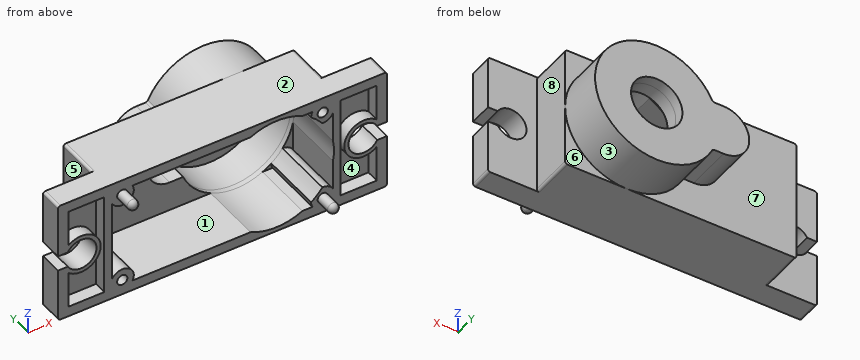
from build123d import *

# Parameters (mm, degrees)
SKETCH1_W            = 22.5
SKETCH1_H            = 12
BOSS_EXTRUDE1_DEPTH  = 6.5
SKETCH2_W            = 22.5
SKETCH2_H            = 12
BOSS_EXTRUDE2_DEPTH  = 0.5
BOSS_EXTRUDE3_DEPTH  = 4.5
SKETCH4_R            = 2.5
BOSS_EXTRUDE4_DEPTH  = 1
CUT_EXTRUDE1_DEPTH   = 7.5
SKETCH6_R            = 3
SKETCH6_R_2          = 2.5
BOSS_EXTRUDE5_DEPTH  = 1.25
BOSS_EXTRUDE7_DEPTH  = 2.25
BOSS_EXTRUDE8_DEPTH  = 1
SKETCH9_R            = 0.625
CUT_EXTRUDE2_DEPTH   = 0.25
SKETCH11_R           = 1.125
SKETCH11_R_2         = 0.5
BOSS_EXTRUDE9_DEPTH  = 6
SKETCH12_R           = 0.5
BOSS_EXTRUDE10_DEPTH = 2
FILLET1_R            = 0.5
FILLET2_R            = 0.25
CUT_EXTRUDE3_DEPTH   = 6


with BuildPart() as part:
    # Sketch1 → Boss-Extrude1 (new body)
    with BuildSketch(Plane(origin=(0, 0, 0), x_dir=(1, 0, 0), z_dir=(0, 1, 0))):
        Rectangle(SKETCH1_W, SKETCH1_H)
        Polygon((10.25, 5), (-10.25, 5), (-10.75, 5), (-10.75, -5), (-10.25, -5), (10.25, -5), (10.75, -5), (10.75, 5), align=None, mode=Mode.SUBTRACT)
    extrude(amount=BOSS_EXTRUDE1_DEPTH)

    # Sketch2 → Boss-Extrude2 (add)
    with BuildSketch(Plane(origin=(0, 6.5, 0), x_dir=(1, 0, 0), z_dir=(0, 1, 0))):
        Rectangle(SKETCH2_W, SKETCH2_H)
    extrude(amount=-BOSS_EXTRUDE2_DEPTH)

    # Sketch3 → Boss-Extrude3 (add)
    with BuildSketch(Plane(origin=(0, 6.5, 0), x_dir=(1, 0, 0), z_dir=(0, 1, 0))):
        with BuildLine():
            Line((-1.25, 2.5), (-0.204356057, 2.5))
            ThreePointArc((-0.204356057, 2.5), (11.25, 0), (-0.204356057, -2.5))
            Line((-0.204356057, -2.5), (-1.25, -2.5))
            ThreePointArc((-1.25, -2.5), (-3.75, 0), (-1.25, 2.5))
        make_face()
        with BuildLine():
            Line((-1.25, 2.1), (0.058661059, 2.1))
            ThreePointArc((0.058661059, 2.1), (10.85, 0), (0.058661059, -2.1))
            Line((0.058661059, -2.1), (-1.25, -2.1))
            ThreePointArc((-1.25, -2.1), (-3.35, 0), (-1.25, 2.1))
        make_face(mode=Mode.SUBTRACT)
    extrude(amount=BOSS_EXTRUDE3_DEPTH)

    # Sketch4 → Boss-Extrude4 (add)
    with BuildSketch(Plane(origin=(0, 11, 0), x_dir=(1, 0, 0), z_dir=(0, 1, 0))):
        with BuildLine():
            ThreePointArc((-1.25, -2.1), (-3.35, 0), (-1.25, 2.1))
            Line((-1.25, 2.1), (0.058661059, 2.1))
            ThreePointArc((0.058661059, 2.1), (10.85, 0), (0.058661059, -2.1))
            Line((0.058661059, -2.1), (-1.25, -2.1))
        make_face()
        with Locations((5.25, 0)):
            Circle(SKETCH4_R, mode=Mode.SUBTRACT)
    extrude(amount=-BOSS_EXTRUDE4_DEPTH)

    # Sketch5 → Cut-Extrude1 (cut, through all)
    with BuildSketch(Plane(origin=(0, 6.5, 0), x_dir=(1, 0, 0), z_dir=(0, 1, 0))):
        with BuildLine():
            Line((-1.25, -2.1), (0.058661059, -2.1))
            ThreePointArc((0.058661059, -2.1), (10.85, 0), (0.058661059, 2.1))
            Line((0.058661059, 2.1), (-1.25, 2.1))
            ThreePointArc((-1.25, 2.1), (-3.35, 0), (-1.25, -2.1))
        make_face()
    extrude(amount=-CUT_EXTRUDE1_DEPTH, mode=Mode.SUBTRACT)

    # Sketch6 → Boss-Extrude5 (add)
    with BuildSketch(Plane.XZ.offset(-10)):
        with Locations((5.25, 0)):
            Circle(SKETCH6_R)
        with Locations((5.25, 0)):
            Circle(SKETCH6_R_2, mode=Mode.SUBTRACT)
    extrude(amount=BOSS_EXTRUDE5_DEPTH)

    # Sketch7 → Boss-Extrude7 (add)
    with BuildSketch(Plane(origin=(0, 0, 0), x_dir=(1, 0, 0), z_dir=(0, 1, 0))):
        with BuildLine():
            Line((-11.25, -6), (-11.25, 6))
            Line((-11.25, 6), (-16, 6))
            Line((-16, 6), (-16, 0.75))
            Line((-16, 0.75), (-15.049038106, 0.75))
            ThreePointArc((-15.049038106, 0.75), (-12.25, 0), (-15.049038106, -0.75))
            Line((-15.049038106, -0.75), (-16, -0.75))
            Line((-16, -0.75), (-16, -6))
            Line((-16, -6), (-11.25, -6))
        make_face()
        with BuildLine():
            Line((-15, 1.430908802), (-15, 5))
            Line((-15, 5), (-11.5, 5))
            Line((-11.5, 5), (-11.5, -5))
            Line((-11.5, -5), (-15, -5))
            Line((-15, -5), (-15, -1.430908802))
            ThreePointArc((-15, -1.430908802), (-11.85, 0), (-15, 1.430908802))
        make_face(mode=Mode.SUBTRACT)
    boss_extrude7 = extrude(amount=BOSS_EXTRUDE7_DEPTH)

    # Sketch8 → Boss-Extrude8 (add)
    with BuildSketch(Plane(origin=(0, 2.25, 0), x_dir=(1, 0, 0), z_dir=(0, 1, 0))):
        with BuildLine():
            Line((-15.049038106, 0.75), (-16, 0.75))
            Line((-16, 0.75), (-16, 6))
            Line((-16, 6), (-11.25, 6))
            Line((-11.25, 6), (-11.25, -6))
            Line((-11.25, -6), (-16, -6))
            Line((-16, -6), (-16, -0.75))
            Line((-16, -0.75), (-15.049038106, -0.75))
            ThreePointArc((-15.049038106, -0.75), (-12.25, 0), (-15.049038106, 0.75))
        make_face()
    boss_extrude8 = extrude(amount=-BOSS_EXTRUDE8_DEPTH)

    # Mirror1: Boss-Extrude7, Boss-Extrude8 across plane
    add(boss_extrude7.mirror(Plane(origin=(0, 0, 0), x_dir=(0, 0, 1), z_dir=(1, 0, 0))))
    add(boss_extrude8.mirror(Plane(origin=(0, 0, 0), x_dir=(0, 0, 1), z_dir=(1, 0, 0))))

    # Sketch9 → Cut-Extrude2 (cut)
    with BuildSketch(Plane.XZ.offset(-10)):
        with Locations((-1.25, 0)):
            Circle(SKETCH9_R)
    extrude(amount=-CUT_EXTRUDE2_DEPTH, mode=Mode.SUBTRACT)

    # Sketch11 → Boss-Extrude9 (add)
    with BuildSketch(Plane.XZ.offset(-6)):
        with Locations((-9.75, 4.5)):
            Circle(SKETCH11_R)
        with Locations((-9.75, -4.5)):
            Circle(SKETCH11_R)
        with Locations((-9.75, -4.5)):
            Circle(SKETCH11_R_2, mode=Mode.SUBTRACT)
        with Locations((9.75, -4.5)):
            Circle(SKETCH11_R)
        with Locations((9.75, 4.5)):
            Circle(SKETCH11_R)
        with Locations((9.75, 4.5)):
            Circle(SKETCH11_R_2, mode=Mode.SUBTRACT)
    extrude(amount=BOSS_EXTRUDE9_DEPTH)

    # Sketch12 → Boss-Extrude10 (add)
    with BuildSketch(Plane.XZ):
        with Locations((-9.75, 4.5)):
            Circle(SKETCH12_R)
        with Locations((9.75, -4.5)):
            Circle(SKETCH12_R)
    extrude(amount=BOSS_EXTRUDE10_DEPTH)

    # Fillet1
    fillet1_edges = [part.edges().sort_by_distance(p)[0] for p in [
        (-10.25, -2, 4.5),
        (9.25, -2, -4.5),
    ]]
    fillet(fillet1_edges, radius=FILLET1_R)

    # Fillet2
    fillet2_edges = [part.edges().sort_by_distance(p)[0] for p in [
        (-16, 1.125, 6),
        (-16, 1.125, -6),
        (16, 1.125, -6),
        (16, 1.125, 6),
        (-0.204356057, 8.75, -2.5),
        (-0.204356057, 8.75, 2.5),
        (-11.25, 4.375, -6),
        (11.25, 4.375, -6),
        (11.25, 4.375, 6),
        (-11.25, 4.375, 6),
    ]]
    fillet(fillet2_edges, radius=FILLET2_R)

    # Sketch13 → Cut-Extrude3 (cut)
    with BuildSketch(Plane.XZ):
        with BuildLine():
            Line((0.058661059, 2.1), (0.058661059, -2.1))
            ThreePointArc((0.058661059, -2.1), (10.85, 0), (0.058661059, 2.1))
        make_face()
    extrude(amount=-CUT_EXTRUDE3_DEPTH, mode=Mode.SUBTRACT)


solid = part.part
Could you check a few things on this model? Use its own coordinates, in mm. Face numbers are marked on the shaded views. A direction names the side the tool comes from. Coordinates: 2 decimals unless noted, no trailing zeros. Write each loop counter-clockwise with the first axis right and the second up, starting at its lowest first coordinate (ties: lowest second). Pieces come first, ordered by that corner, then holes. Notation, with made-up numbers: M 43.5,35.5 L 87.5,35.5 A4 ccw 87.5,42.5 Z; hole C 28.25,-25.5 d9. An arc over 180 degrees is marked long. One line per question, with ' | ' between items.
1) I need wall thicknesses on probe 1 along X at (y, z) = (2.45, -4.5) (3 decimals); probe 2 along X at (y, z) = (3.25, -4.25); probe 3 along Z at (x, y) = (1.5, 2.25). Which ranges of each line are inside material? Lowest first, please. Write a range as [from, to].
Checks:
probe 1: [-11.25, -10.25], [-9.25, -8.625], [8.625, 11.25] | probe 2: [-11.25, -10.18], [-9.32, -8.65], [8.9, 11.25] | probe 3: [-6, -5], [5, 6]
2) Imagine slicing it at D-D, the plane x = -9.75. Write out the boundary of the cut face in (y, z) (3 decimals), and give its area (3 significant figures).
Checks:
outline: M -1.5,4 L 0,4 L 0,3.375 L 6,3.375 L 6,-3.375 L 0,-3.375 L 0,-4 L 6,-4 L 6,-5 L 0,-5 L 0,-6 L 6.5,-6 L 6.5,6 L 0,6 L 0,5 L -1.5,5 A0.5 ccw Z | area: 33.4 mm²
3) Imagine slicing it at A-A, the plane x = -13.75. Write out the boundary of the cut face in (y, z).
Checks:
outline: M 0,-6 L 2.25,-6 L 2.25,-1.5 L 0,-1.5 L 0,-1.9 L 1.25,-1.9 L 1.25,-5 L 0,-5 Z; M 0,1.5 L 2.25,1.5 L 2.25,6 L 0,6 L 0,5 L 1.25,5 L 1.25,1.9 L 0,1.9 Z
4) For the marked faces 4, 5, 6, 7 and 8, which set-ups out of +Z, -Z, +X, -X, +Y, -Y let a thin tool reach every point of the face, with its end or its side?
Checks:
face 4: -Y | face 5: +Z, -Z, -X, +Y | face 6: -Z, +X, +Y | face 7: -X, +Y | face 8: +Z, -Z, +X, +Y
5) If we mould it in two halves opening along Z, with no side actions, what happens to the marked faces 1, 2 and 3? For each: released by +Z, released by -Z, zero draft, split by the parting line, or undercut.
Checks:
face 1: undercut | face 2: released by +Z | face 3: split by the parting line
6) Imagine slicing it at B-B, the plane y = 7. Write out the boundary of the cut face in (x, z), and give its area (3 significant figures).
Checks:
outline: M -1.25,-2.5 L -0.36,-2.5 A0.25 cw -0.14,-2.64 A6 ccw long -0.14,2.64 A0.25 cw -0.36,2.5 L -1.25,2.5 A2.5 ccw Z; hole M -1.25,-2.1 L 0.06,-2.1 A5.6 ccw long 0.06,2.1 L -1.25,2.1 A2.1 ccw Z | area: 16.5 mm²
7) For pin 1 Ø5 at (x, z) = (5.5, 3) entering from -Y; pin 2 Ø5 at (x, z) = (7.5, -3.5) entering from -Y; pin 3 Ø0.8 at (x, z) = (-1.25, 0) entering from -Y; pin 4 Ø3.5 at (x, z) = (13.75, 0) entering from +Y, each with a flat end and sliding along its axis, tell me the tip position at first contact or that it passes through.
Checks:
pin 1: y = 8.75 | pin 2: y = -2 | pin 3: y = 10.25 | pin 4: y = 2.25
8) Imagine slicing it at C-C, the plane y = -1. Write out the boundary of the cut face in (x, z), and give its area (3 significant figures).
Checks:
outline: C -9.75,4.5 d1; C 9.75,-4.5 d1 | area: 1.57 mm²
